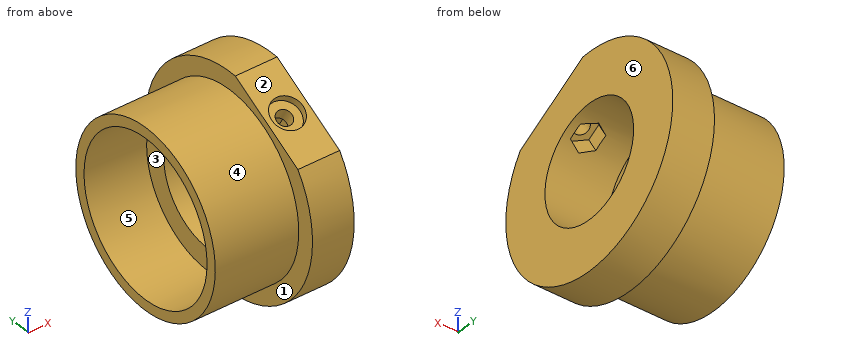
from build123d import *

# Parameters (mm, degrees)
SKETCH147_W          = 50.8
SKETCH147_H          = 7
POCKET092_DEPTH      = 30.001
POCKET092_DEPTH_BACK = 6.001
SKETCH144_R          = 2.2
POCKET093_DEPTH      = 41.528172
POCKET094_DEPTH      = 21.15
SKETCH148_R          = 4.5
POCKET095_DEPTH      = 5


with BuildPart() as part:
    # Sketch143 → Revolution004 (revolve)
    with BuildSketch(Plane.XZ):
        Polygon((0, 25.4), (0, 30.4), (12, 30.4), (12, 16.15), (-6, 16.15), (-6, 22.4), (-24, 22.4), (-24, 25.4), align=None)
    revolve(axis=Axis((0, 0, 0), (1, 0, 0)))

    # Sketch147 (on DatumPlane) → Pocket092 (cut, two sides)
    with BuildSketch(Plane(origin=(6, 0, 0), x_dir=(0, -0.866025, -0.5), z_dir=(1, 0, 0))) as pocket092_sk:
        with Locations((0, -30.9)):
            Rectangle(SKETCH147_W, SKETCH147_H)
    extrude(amount=-POCKET092_DEPTH, mode=Mode.SUBTRACT)
    extrude(pocket092_sk.sketch, amount=POCKET092_DEPTH_BACK, mode=Mode.SUBTRACT)

    # Sketch144 (on DatumPlane) → Pocket093 (cut, through all)
    with BuildSketch(Plane(origin=(6, 0, 0), x_dir=(1, 0, 0), z_dir=(0, 0.5, -0.866025))):
        Circle(SKETCH144_R)
    extrude(amount=-POCKET093_DEPTH, mode=Mode.SUBTRACT)

    # Sketch145 (on DatumPlane) → Pocket094 (cut)
    with BuildSketch(Plane(origin=(6, 0, 0), x_dir=(1, 0, 0), z_dir=(0, 0.5, -0.866025))):
        Polygon((3.65, -2.107328), (3.65, 2.107328), (0, 4.214657), (-3.65, 2.107328), (-3.65, -2.107328), (0, -4.214657), align=None)
    extrude(amount=-POCKET094_DEPTH, mode=Mode.SUBTRACT)

    # Sketch148 (on DatumPlane) → Pocket095 (cut)
    with BuildSketch(Plane(origin=(6, -12.575, 21.780539), x_dir=(1, 0, 0), z_dir=(0, 0.5, -0.866025))):
        Circle(SKETCH148_R)
    extrude(amount=-POCKET095_DEPTH, mode=Mode.SUBTRACT)


with BuildPart() as part_1:
    # Body022029 placement: moved
    add(part.part.moved(Location((194, 0, 834))))


solid = part_1.part
Part model, mm, in its own coordinate system. Face numbers are marked on the shaded views. A direction names the side the tool comes from. Give positions to 0.01 mm unless a question says otherwise; leave off trailing zeros. Order: outer loops, then holes, each group sorted by start corner. A loop starts at its lowest first (then second) coordinate and runs counter-clockwise, first axis right, second up. Notation, with made-up numbers: (30.25, 42.5) - (82.25, 42.5) arc R21 ccw to (82.25, 58.5) - close; hole circle Ø9 at (22.25, 70). An arc over 180 degrees is marked (long way). One line per question, with ' | ' between items.
1. Band-saw the part on A-A on z = 834. List the corners of the cut face in (x, y).
Filled in:
outline: (170, -25.4) - (194, -25.4) - (194, -30.4) - (206, -30.4) - (206, -16.15) - (188, -16.15) - (188, -22.4) - (170, -22.4) - close; (170, 22.4) - (188, 22.4) - (188, 16.15) - (206, 16.15) - (206, 30.4) - (194, 30.4) - (194, 25.4) - (170, 25.4) - close
2. Pull direction Z, two halves, no side cores. Call the marked faces 3, 4, 5 and 6: +Z half, -Z half, draft (parallel to the pull), parting line (faces both ways), or undercut.
Filled in:
face 3: undercut | face 4: parting line | face 5: undercut | face 6: draft
3. Band-saw the part on B-B on y = 0. List the corners of the cut face in (x, z).
Filled in:
outline: (170, 808.6) - (194, 808.6) - (194, 803.6) - (206, 803.6) - (206, 817.85) - (188, 817.85) - (188, 811.6) - (170, 811.6) - close; (170, 856.4) - (188, 856.4) - (188, 850.15) - (206, 850.15) - (206, 864.4) - (194, 864.4) - (194, 859.4) - (170, 859.4) - close
4. Which spindle directions (+Z, -Z, +X, -X, +Y, -Y) get a long thin tool onto all of the face, cutting with end or side? Do the marked faces 1 and 2. Say none if no direction does.
Filled in:
face 1: -X | face 2: +Z, +X, -X, -Y
5. Band-saw the part on C-C on x = 187. List the corners of the cut face in (y, z), then the cut area to 3 significant figures.
Filled in:
outline: circle Ø50.8 at (0, 834); hole circle Ø44.8 at (0, 834) | area: 451 mm²
6. Band-saw the part on D-D on y = 20.5. List the corners of the cut face in (x, z).
Filled in:
outline: (170, 819) - (194, 819) - (194, 811.55) - (206, 811.55) - (206, 856.45) - (194, 856.45) - (194, 849) - (170, 849) - (170, 843.03) - (188, 843.03) - (188, 824.97) - (170, 824.97) - close
7. Drop flat-ended pins along their axis: P1, Ø8, axis at y = -10.5, z = 839.5, coming from the +X side; P2, Ø6, axis at x = 174, z = 819, coming from the +Y side; P3, Ø3, axis at x = 200, y = -18.5, coming from the +Z side; P4, Ø2, axis at x = 200, z = 845, coming from the +Y side. Give the stop position or say it passes through.
Filled in:
P1: through | P2: y = 22.39 | P3: z = 855.55 | P4: y = 28.71
8. Drill centre lines: probe 1 along Z at (x, y) = (179.5, 0); probe 2 along Y at (x, z) = (180.75, 834); probe 3 along Y at (x, z) = (196, 834). Where is each one in solid material? Low to high.
Filled in:
probe 1: 808.6 to 811.6, 856.4 to 859.4 | probe 2: -25.4 to -22.4, 22.4 to 25.4 | probe 3: -30.4 to -16.15, 16.15 to 30.4
